Check sheet for the drawn part. Datum: minimum x, y, z corner. Units: mm. A direction names the side the tool comes from. Round coordinates to 2 decimals unless told otherwise and drop trailing zeros. Write each loop counter-clockwise with the first axis right and the second up, starting at its lowest first coordinate (ties: lowest second). Pieces come first, ordered by that corner, then holes.
Item 1: Cross-section at C-C on z = 3.5. Enter the section's corners in (x, y), plus the area to 3 significant figures.
Item 2: Cross-section at B-B on x = 30. Enter the section's corners in (y, z).
Item 3: Material ranges on line 1 (Y direction, x = 14.5, z = 0.7); line 2 (Y direction, x = 45.5, z = 4.85); line 3 (Y direction, x = 30, z = 2.75), recorded low to high.
Item 4: Tool access check on the marked faces 3 and 4. Record the directions out of +Z, -Z, +X, -X, +Y, -Y that give a thin tool (end or side, any length) a straight path to the whole face; none if there is none.
Item 5: Go/stop test with flat-tipped pins: pin 1 Ø10 at (x, z) = (51.5, 21.5) entering from -Y; pin 2 Ø6.5 at (x, y) = (15, 12.5) entering from +Z; pin 3 Ø1.8 at (y, z) = (57.5, 13) entering from -X. Record where each tip stops, or that it passes through.
Item 6: Cross-section at D-D on z = 15. Enter the section's corners in (x, y).
Item 7: Cross-section at A-A on y = 45. Enter the section's corners in (x, z), plus the area to 3 significant figures.
Item 8: Release check for a two-part mould opening along X. For the marked faces 1 and 2 record: +X half, -X half, draft (parallel to the pull), parting line (faces both ways), or undercut.
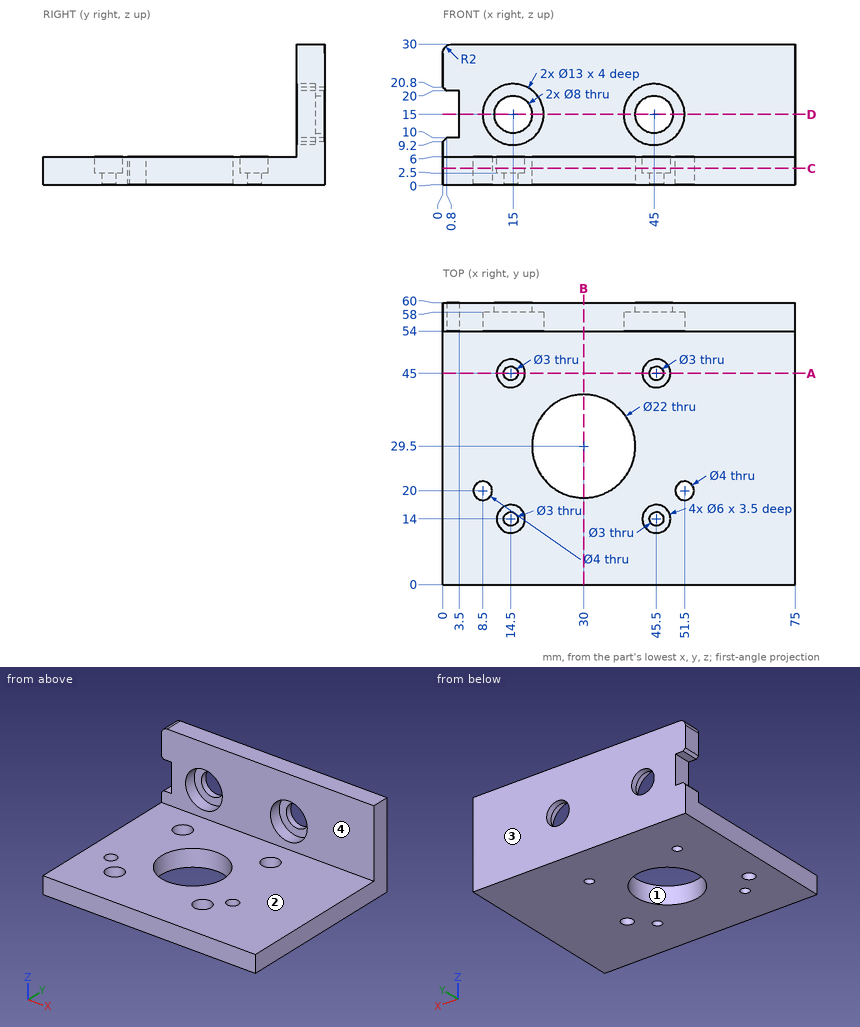
Response values:
1. outline: (0, 0) - (75, 0) - (75, 60) - (0, 60) - close; hole circle Ø4 at (8.5, 20); hole circle Ø6 at (14.5, 14); hole circle Ø6 at (14.5, 45); hole circle Ø22 at (30, 29.5); hole circle Ø6 at (45.5, 14); hole circle Ø6 at (45.5, 45); hole circle Ø4 at (51.5, 20)
1. area: 3,980 mm2
2. outline: (0, 0) - (18.5, 0) - (18.5, 6) - (0, 6) - close; (40.5, 0) - (60, 0) - (60, 30) - (54, 30) - (54, 6) - (40.5, 6) - close
3. line 1: y = 0 to 12.5, 15.5 to 43.5, 46.5 to 60
3. line 2: y = 0 to 11, 17 to 42, 48 to 60
3. line 3: y = 0 to 18.5, 40.5 to 60
4. face 3: +Z, -Z, +X, -X, +Y
4. face 4: +Z, +X, -X, -Y
5. pin 1: stops at y = 54
5. pin 2: stops at z = 6
5. pin 3: stops at x = 3.5
6. outline: (3.5, 54) - (8.5, 54) - (8.5, 58) - (11, 58) - (11, 60) - (3.5, 60) - close; (19, 58) - (21.5, 58) - (21.5, 54) - (38.5, 54) - (38.5, 58) - (41, 58) - (41, 60) - (19, 60) - close; (49, 58) - (51.5, 58) - (51.5, 54) - (75, 54) - (75, 60) - (49, 60) - close
7. outline: (0, 0) - (13, 0) - (13, 2.5) - (11.5, 2.5) - (11.5, 6) - (0, 6) - close; (16, 0) - (44, 0) - (44, 2.5) - (42.5, 2.5) - (42.5, 6) - (17.5, 6) - (17.5, 2.5) - (16, 2.5) - close; (47, 0) - (75, 0) - (75, 6) - (48.5, 6) - (48.5, 2.5) - (47, 2.5) - close
7. area: 393 mm2
8. face 1: undercut
8. face 2: draft
